Verification items for the finished model (mm, model axes). Coordinates: 2 decimals unless noted, no trailing zeros. Order: outer loops, then holes, each group sorted by start corner. A loop starts at its lowest first (then second) coordinate and runs counter-clockwise, first axis right, second up. Notation, with made-up numbers: (-18.5, 89) -> (-9.5, 89) arc R9 ccw to (-9.5, 105) -> close; hole circle Ø6 at (46, 1.5). An arc over 180 degrees is marked (long way). Answer as CSV lines item,"result".
```python
from build123d import *

# Parameters (mm, degrees)
SKETCH1_W                = 50
SKETCH1_H                = 6
BOSS_EXTRUDE1_DEPTH      = 40
BOSS_EXTRUDE1_DEPTH_BACK = 46
SKETCH2_R                = 3.3
CUT_EXTRUDE1_DEPTH       = 7
FILLET1_R                = 10


with BuildPart() as part:
    # Sketch1 → Boss-Extrude1 (new body, two sides)
    with BuildSketch(Plane.XY) as boss_extrude1_sk:
        with Locations((371.231060123, 22)):
            Rectangle(SKETCH1_W, SKETCH1_H)
    extrude(amount=BOSS_EXTRUDE1_DEPTH)
    extrude(boss_extrude1_sk.sketch, amount=-BOSS_EXTRUDE1_DEPTH_BACK)

    # Sketch2 → Cut-Extrude1 (cut, through all)
    with BuildSketch(Plane.XZ.offset(-19)):
        with Locations((371.231060123, -26)):
            Circle(SKETCH2_R)
        with Locations((371.231060123, 20)):
            Circle(SKETCH2_R)
    extrude(amount=-CUT_EXTRUDE1_DEPTH, mode=Mode.SUBTRACT)

    # Fillet1
    fillet1_edges = [part.edges().sort_by_distance(p)[0] for p in [
        (396.231060123, 22, -46),
        (346.231060123, 22, 40),
        (396.231060123, 22, 40),
        (346.231060123, 22, -46),
    ]]
    fillet(fillet1_edges, radius=FILLET1_R)


solid = part.part
```
Item 1: Depth check by flat-ended pin: pin 1 Ø7.5 at (x, z) = (371.23, -26) entering from +Y; pin 2 Ø1.5 at (x, y) = (352.5, 24) entering from -Z; pin 3 Ø3 at (x, z) = (372, 19) entering from -Y (1 decimal). Enter the tip coordinate at first touch or a pass-through.
Answer list:
pin 1,"y = 25"
pin 2,"z = -45.55"
pin 3,"through"
Item 2: Thickness scan on line 1 (Z direction, x = 373.5, y = 21.6); line 2 (Z direction, x = 387, y = 20.3); line 3 (X direction, y = 23.05, z = 19). Record the ranges inside material, lowest first.
Answer list:
line 1,"-46 to -28.4, -23.6 to 17.6, 22.4 to 40"
line 2,"-45.97 to 39.97"
line 3,"346.23 to 368.09, 374.38 to 396.23"
Item 3: Release check for a two-part mould opening along X. For faces 1 (the flat face through (371, 19, -2)), 2 (the cylindrical face through (367.934, 21.958, 20.145)), 3 (the cylindrical face through (393.22, 22.04, -43.15)), 4 (the cylindrical face through (349.08, 22.04, 36.99)) record: +X half, -X half, draft (parallel to the pull), parting line (faces both ways), or undercut.
Answer list:
face 1,"draft"
face 2,"undercut"
face 3,"+X half"
face 4,"-X half"
Item 4: Section check A-A, the plane z = 20. Record the boundary of the cut face in (x, y).
Answer list:
outline,"(346.23, 19) -> (367.93, 19) -> (367.93, 25) -> (346.23, 25) -> close; (374.53, 19) -> (396.23, 19) -> (396.23, 25) -> (374.53, 25) -> close"
Item 5: Section check C-C, the plane x = 351.5. Record the boundary of the cut face in (y, z), plus the area to 3 significant figures.
Answer list:
outline,"(19, -44.81) -> (25, -44.81) -> (25, 38.81) -> (19, 38.81) -> close"
area,"502 mm2"
Item 6: Section check B-B, the plane y = 20.1. Record the boundary of the cut face in (x, z), plus the area to 3 significant figures.
Answer list:
outline,"(346.23, -36) arc R10 ccw to (356.23, -46) -> (386.23, -46) arc R10 ccw to (396.23, -36) -> (396.23, 30) arc R10 ccw to (386.23, 40) -> (356.23, 40) arc R10 ccw to (346.23, 30) -> close; hole circle Ø6.6 at (371.23, -26); hole circle Ø6.6 at (371.23, 20)"
area,"4,150 mm2"
